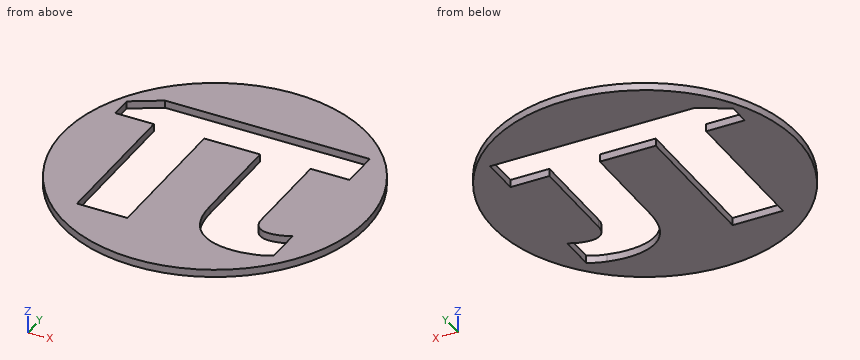
```python
from build123d import *

# Parameters (mm, degrees)
F0_R     = 40
F1_DEPTH = 2


with BuildPart() as f1:
    # F0 (on Top) → F1 (new body)
    with BuildSketch(Plane.XY):
        Circle(F0_R)
        with BuildLine():
            add(Edge.make_bspline(
                [(19.3472222222, -14.6533066589), (20.5208333333, -15.7227511033), (22.2569444444, -15.7227511033)],
                knots=[0, 0, 0, 1, 1, 1], degree=2))
            add(Edge.make_bspline(
                [(22.2569444444, -15.7227511033), (25.1597222222, -15.7227511033), (27.8958333333, -14.1949733256)],
                knots=[0, 0, 0, 1, 1, 1], degree=2))
            Line((27.8958333333, -14.1949733256), (27.8958333333, -23.7088622145))
            add(Edge.make_bspline(
                [(27.8958333333, -23.7088622145), (26.1180555556, -24.7921955478), (23.3611111111, -25.4449733256)],
                knots=[0, 0, 0, 1, 1, 1], degree=2))
            add(Edge.make_bspline(
                [(23.3611111111, -25.4449733256), (20.6041666667, -26.0977511033), (18.2569444444, -26.0977511033)],
                knots=[0, 0, 0, 1, 1, 1], degree=2))
            add(Edge.make_bspline(
                [(18.2569444444, -26.0977511033), (11.7430555556, -26.0977511033), (8.3402777778, -22.5352511033)],
                knots=[0, 0, 0, 1, 1, 1], degree=2))
            add(Edge.make_bspline(
                [(8.3402777778, -22.5352511033), (4.9375, -18.9727511033), (4.9375, -11.9033066589)],
                knots=[0, 0, 0, 1, 1, 1], degree=2))
            Line((4.9375, -11.9033066589), (4.9375, 13.1939155633))
            Line((4.9375, 13.1939155633), (-9.7430555556, 13.1939155633))
            Line((-9.7430555556, 13.1939155633), (-9.7430555556, -25.2227511033))
            Line((-9.7430555556, -25.2227511033), (-22.9791666667, -25.2227511033))
            Line((-22.9791666667, -25.2227511033), (-22.9791666667, 13.1939155633))
            Line((-22.9791666667, 13.1939155633), (-33.0902777778, 13.1939155633))
            Line((-33.0902777778, 13.1939155633), (-33.0902777778, 18.8744711189))
            Line((-33.0902777778, 18.8744711189), (-25.3680555556, 23.3050266744))
            Line((-25.3680555556, 23.3050266744), (28.4097222222, 23.3050266744))
            Line((28.4097222222, 23.3050266744), (28.4097222222, 13.1939155633))
            Line((28.4097222222, 13.1939155633), (18.1736111111, 13.1939155633))
            Line((18.1736111111, 13.1939155633), (18.1736111111, -11.3755288811))
            add(Edge.make_bspline(
                [(18.1736111111, -11.3755288811), (18.1736111111, -13.5838622145), (19.3472222222, -14.6533066589)],
                knots=[0, 0, 0, 1, 1, 1], degree=2))
        make_face(mode=Mode.SUBTRACT)
    extrude(amount=F1_DEPTH)


solid = f1.part
```
Part model, mm, in its own coordinate system. Give positions to 0.01 mm unless a question says otherwise; leave off trailing zeros. Write each loop counter-clockwise with the first axis right and the second up, starting at its lowest first coordinate (ties: lowest second). Pieces come first, ordered by that corner, then holes. Notation, with made-up numbers: (58, 86.5) -> (102, 86.5) arc R25 cw to (102, 111.5) -> close; hole circle Ø5 at (56.25, 22.25). An arc over 180 degrees is marked (long way). Put each result on its own line as item: value. Start each with the question number.
Item 1: Cut at C-C (x = -19). List the corners of the cut face in (y, z), then the cut area to 3 significant figures.
Item 2: Pin check, flat tips, straight feed: pin 1 Ø0.6 at (y, z) = (5.5, 1.5) entering from +X; pin 2 Ø1 at (y, z) = (-20.5, 1.5) entering from -X; pin 3 Ø1 at (y, z) = (19, 1) entering from -X. Stop position of each tip, or through.
Item 3: Wall check: L1, parallel to X at y = -21, z = 0.2; L2, parallel to X at y = -12.5, z = 0.1; L3, parallel to Y at x = 0, z = 1.8. Give the ranges that are in metal, low to high. Write a range as [from, to].
Item 4: Cut at D-D (x = 25). State how many separate pieces and enclosed holes the cut face has, then the cut area to 3 significant figures.
Item 5: Cut at B-B (y = 0). List the corners of the cut face in (x, z).
Item 6: Cut at A-A (x = 0). List the corners of the cut face in (y, z), then the cut area to 3 significant figures.
Answer list:
1. outline: (-35.2, 0) -> (-25.22, 0) -> (-25.22, 2) -> (-35.2, 2) -> close; (23.31, 0) -> (35.2, 0) -> (35.2, 2) -> (23.31, 2) -> close
1. area: 43.7 mm2
2. pin 1: stops at x = 39.66
2. pin 2: stops at x = -34.64
2. pin 3: stops at x = -35.46
3. L1: x = [-34.04, -22.98], [-9.74, 7.13], [27.9, 34.04]
3. L2: x = [-38, -22.98], [-9.74, 4.94], [18.26, 38]
3. L3: y = [-40, 13.19], [23.31, 40]
4. separate pieces: 3
4. enclosed holes: 0
4. area: 85.4 mm2
5. outline: (-40, 0) -> (-22.98, 0) -> (-22.98, 2) -> (-40, 2) -> close; (-9.74, 0) -> (4.94, 0) -> (4.94, 2) -> (-9.74, 2) -> close; (18.17, 0) -> (40, 0) -> (40, 2) -> (18.17, 2) -> close
6. outline: (-40, 0) -> (13.19, 0) -> (13.19, 2) -> (-40, 2) -> close; (23.31, 0) -> (40, 0) -> (40, 2) -> (23.31, 2) -> close
6. area: 140 mm2
